CAD build for the part. Positions are in the model's coordinates, mm. Face numbers are marked on the shaded views. A direction names the side the tool comes from. Round coordinates to 2 decimals unless told otherwise and drop trailing zeros. Loops run counter-clockwise (first coordinate to the right, second up) from the corner with the lowest first, then second, coordinate; pieces in that order, holes last. Notation, with made-up numbers: M -11,-6 L 9,-6 A36 cw 9,30 Z; hole C 70.5,11.5 d5. An arc over 180 degrees is marked long. One line per item, written item: value. Start each with the question number.
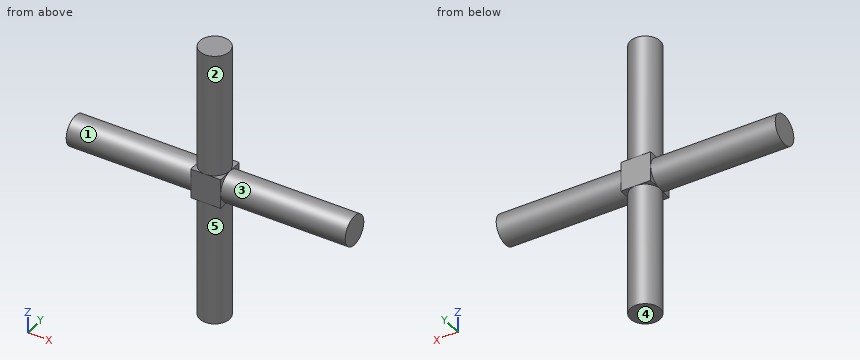
from build123d import *

# Parameters (mm, degrees)
SKETCH1_W           = 1.5
SKETCH1_H           = 1.5
BOSS_EXTRUDE1_DEPTH = 1.5
SKETCH3_R           = 0.75
BOSS_EXTRUDE2_DEPTH = 7
SKETCH4_R           = 0.75
BOSS_EXTRUDE3_DEPTH = 7


with BuildPart() as part:
    # Sketch1 → Boss-Extrude1 (new body)
    with BuildSketch(Plane(origin=(0, 0, 0), x_dir=(1, 0, 0), z_dir=(0, 1, 0))):
        Rectangle(SKETCH1_W, SKETCH1_H)
    extrude(amount=BOSS_EXTRUDE1_DEPTH)

    # Sketch3 → Boss-Extrude2 (add, symmetric)
    with BuildSketch(Plane(origin=(0, 0, 0), x_dir=(0, 0, -1), z_dir=(1, 0, 0))):
        with Locations((0, 0.75)):
            Circle(SKETCH3_R)
    extrude(amount=BOSS_EXTRUDE2_DEPTH, both=True)

    # Sketch4 → Boss-Extrude3 (add, symmetric)
    with BuildSketch(Plane.XY):
        with Locations(Location((-0.013990229, 0.75, 0), (0, 0, 191.084007893))):
            Circle(SKETCH4_R)
    extrude(amount=BOSS_EXTRUDE3_DEPTH, both=True)


solid = part.part
(1) Slice it at B-B, the plane z = -0.5. List the corners of the cut face in (x, y), and give its area (3 significant figures).
(2) Probe L1, parallel to Z at x = -5.5, y = 0.6; L2, parallel to X at y = 0.8, z = -4; L3, parallel to X at y = 1.1, z = 6.75. List the from-to ranges inside material, lowest first.
(3) Slice it at C-C, the plane x = -5. List the corners of the cut face in (y, z).
(4) Which spindle directions (+Z, -Z, +X, -X, +Y, -Y) get a long thin tool onto all of the face, cutting with end or side? Do the marked faces 1, 2, 3, 4 and 5. Say none if no direction does.
(5) Slice it at A-A, the plane y = 1.25. List the corners of the cut face in (x, z).
(6) Flat gauge pin, fed straight in: P1, Ø4, axis at x = 5, z = 3.5, coming from the -Y side. Where does the tip first touch, or does it go through?
(7) Slice it at D-D, the plane y = 0.2. List the corners of the cut face in (x, z), and give its area (3 significant figures).
Check result:
1. outline: M -7,0.19 L -0.75,0.19 L -0.75,0 L 0.75,0 L 0.75,0.19 L 7,0.19 L 7,1.31 L 0.75,1.31 L 0.75,1.5 L -0.75,1.5 L -0.75,1.31 L -7,1.31 Z
1. area: 16.2 mm^2
2. L1: z = -0.73 to 0.73
2. L2: x = -0.76 to 0.73
2. L3: x = -0.68 to 0.65
3. outline: C 0.75,0 d1.5
4. face 1: -X
4. face 2: +Z
4. face 3: +X
4. face 4: -Z, +X, -X, +Y, -Y
4. face 5: -Z
5. outline: M -7,-0.56 L -0.75,-0.56 L -0.75,-0.75 L -0.57,-0.75 L -0.57,-7 L 0.55,-7 L 0.55,-0.75 L 0.75,-0.75 L 0.75,-0.56 L 7,-0.56 L 7,0.56 L 0.75,0.56 L 0.75,0.75 L 0.55,0.75 L 0.55,7 L -0.57,7 L -0.57,0.75 L -0.75,0.75 L -0.75,0.56 L -7,0.56 Z
6. P1: passes through
7. outline: M -7,-0.51 L -0.75,-0.51 L -0.75,-0.75 L -0.52,-0.75 L -0.52,-7 L 0.5,-7 L 0.5,-0.75 L 0.75,-0.75 L 0.75,-0.51 L 7,-0.51 L 7,0.51 L 0.75,0.51 L 0.75,0.75 L 0.5,0.75 L 0.5,7 L -0.52,7 L -0.52,0.75 L -0.75,0.75 L -0.75,0.51 L -7,0.51 Z
7. area: 27.7 mm^2
